Geometry: see drawing. Coordinates: mm, zero at the bounding-box minimum. A direction names the side the tool comes from. Coordinates: 2 decimals unless noted, no trailing zeros. Write each loop counter-clockwise with the first axis right and the second up, starting at its lowest first coordinate (ties: lowest second). Pieces come first, ordered by that corner, then holes. Notation, with made-up numbers: M 79.25,-7.5 L 121.25,-7.5 A25 ccw 121.25,26.5 Z; hole C 19,-19.5 d10. An arc over 180 degrees is marked long. Write item = value, one per line. Start each with the question number.
1. Pull-direction query (Y, two-part tool) for the marked faces 3, 4 and 5; classes: pulls with the +Y half, pulls with the -Y half, needs draft (parallel to the pull), parting line crosses it, or undercut.
2. Pin query (flat end, axial travel): pin 1 Ø4 at (x, y) = (45, 13.5) entering from +Z; pin 2 Ø3.5 at (x, z) = (74.93, 5.08) entering from +Y; pin 3 Ø1 at (x, y) = (57.5, 31) entering from -Z; pin 4 Ø10 at (x, y) = (36.5, 29.5) entering from -Z. Return the tip coordinate at first contact, or that it passes through.
3. Line query: line 1 along X through (y, z) = (16.5, 40) (1 decimal); line 2 along Y through (x, z) = (12.5, 74); line 3 along X through (y, z) = (31, 48.5). Output: solid intervals per line, ascending.
4. Section query D-D (x = 70). Output: boundary loops of the cut face in (y, z).
5. Access query for the marked faces 1 and 2. Directions: +Z, -Z, +X, -X, +Y, -Y. A direction counts if a zero-diameter tool reaches every point of the face in a straight line with its end or side. Return the directions, or none.
6. Section query B-B (x = 5.08). Give the number of separate pieces and of enclosed holes in the cut face.
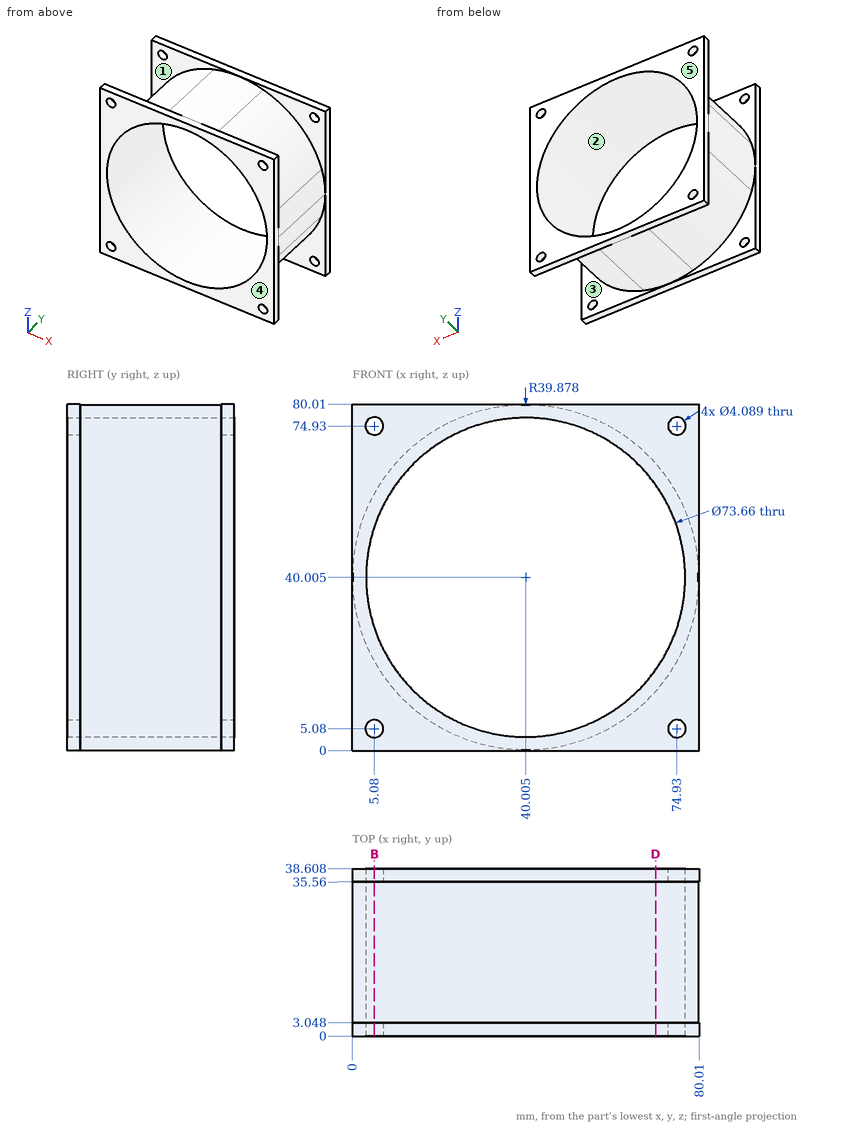
Results are:
q1.face_3 = undercut
q1.face_4 = pulls with the -Y half
q1.face_5 = pulls with the +Y half
q2.pin_1 = 79.77
q2.pin_2 = through
q2.pin_3 = 3.93
q2.pin_4 = 0.13
q3.line_1 = 0.1 to 3.2, 76.8 to 79.9
q3.line_2 = 0 to 3.05, 35.56 to 38.61
q3.line_3 = 1.04 to 4.17, 75.84 to 78.97
q4.outline = M 0,0 L 3.05,0 L 3.05,13.73 L 35.56,13.73 L 35.56,0 L 38.61,0 L 38.61,18.63 L 0,18.63 Z; M 0,61.38 L 38.61,61.38 L 38.61,80.01 L 35.56,80.01 L 35.56,66.28 L 3.05,66.28 L 3.05,80.01 L 0,80.01 Z
q5.face_1 = none
q5.face_2 = +Y, -Y
q6.separate_pieces = 6
q6.enclosed_holes = 0
